```python
from build123d import *

# Parameters (mm, degrees)
F0_W      = 127
F0_H      = 76.2
F1_DEPTH  = 6.35
F3_DEPTH  = 6.35
F5_DEPTH  = 6.35
F7_DEPTH  = 6.35
F9_DEPTH  = 6.35
F11_DEPTH = 6.35
F13_DEPTH = 6.35


with BuildPart() as f1:
    # F0 (on Top) → F1 (new body)
    with BuildSketch(Plane.XY):
        with Locations((63.5, -38.1)):
            Rectangle(F0_W, F0_H)
    extrude(amount=F1_DEPTH)

    # F2 (on face) → F3 (cut, through all)
    with BuildSketch(Plane.XY.offset(6.35)):
        with BuildLine():
            ThreePointArc((8.986218, -38.1), (5.353199, -34.466981), (1.72018, -38.1))
            ThreePointArc((1.72018, -38.1), (5.353199, -41.733019), (8.986218, -38.1))
        make_face()
    extrude(amount=-F3_DEPTH, mode=Mode.SUBTRACT)

    # F4 (on face) → F5 (join)
    with BuildSketch(Plane.XY.offset(6.35)):
        with BuildLine():
            ThreePointArc((11.837447, -76.2), (35.286069, -38.1), (11.837447, 0))
            Line((11.837447, 0), (11.837447, -76.2))
        make_face()
    extrude(amount=F5_DEPTH)

    # F6 (on face) → F7 (cut)
    with BuildSketch(Plane.XY.offset(12.7)):
        with BuildLine():
            ThreePointArc((14.233802, -68.477303), (30.151871, -37.113268), (14.233802, -5.749233))
            Line((14.233802, -5.749233), (14.233802, -68.477303))
        make_face()
    extrude(amount=-F7_DEPTH, mode=Mode.SUBTRACT)

    # F8 (on face) → F9 (join)
    with BuildSketch(Plane.XY.offset(6.35)):
        Polygon((81.754573, -76.2), (51.588718, 0), (26.779415, -76.2), (36.64675, -76.2), (47.923706, -40.566836), (59.482586, -40.566836), (69.418724, -76.2), align=None)
        Polygon((45.034298, -35.888964), (51.588718, -15.757531), (59.341624, -35.888964), align=None, mode=Mode.SUBTRACT)
    extrude(amount=F9_DEPTH)

    # F10 (on face) → F11 (join)
    with BuildSketch(Plane.XY.offset(6.35)):
        with BuildLine():
            Line((84.432848, 0), (84.432848, -76.2))
            ThreePointArc((84.432848, -76.2), (115.125997, -38.1), (84.432848, 0))
        make_face()
        with BuildLine():
            Line((88.097863, -69.604993), (88.097863, -7.158854))
            ThreePointArc((88.097863, -7.158854), (109.621547, -38.381923), (88.097863, -69.604993))
        make_face(mode=Mode.SUBTRACT)
    extrude(amount=F11_DEPTH)

    # F12 (on face) → F13 (join)
    with BuildSketch(Plane.XY.offset(6.35)):
        with BuildLine():
            ThreePointArc((119.378194, -66.891998), (116.194297, -64.889157), (113.354176, -67.355387))
            Line((113.354176, -67.355387), (119.223736, -74.769571))
            Line((119.223736, -74.769571), (124.320991, -66.891998))
            ThreePointArc((124.320991, -66.891998), (121.849593, -64.724744), (119.378194, -66.891998))
        make_face()
    extrude(amount=F13_DEPTH)


solid = f1.part
```
Source: CAD feature listing. Evaluate the final solid. Frame: model axes, mm. A direction names the side the tool comes from. Coordinates: 2 decimals unless noted, no trailing zeros. Loops run counter-clockwise (first coordinate to the right, second up) from the corner with the lowest first, then second, coordinate; pieces in that order, holes last. Notation, with made-up numbers: (67.25, -30) -> (83.25, -30) arc R9 cw to (83.25, -25) -> close; hole circle Ø7 at (79.25, 86.5). An arc over 180 degrees is marked (long way). One line per item, written item: value. Start each with the question number.
Q1. Section query A-A, the plane y = -38.1. Return the cut outline in (x, z).
Q2. Line query: line 1 along X through (y, z) = (-38.1, 2); line 2 along X through (y, z) = (-59, 8.5); line 3 along X through (y, z) = (-30.5, 11). Output: solid intervals per line, ascending.
Q3. Mould query, pull axis Y, two halves, no side actions, for faces 5 (the face through (127, -39, 3)), 6 (the face through (63, 0, 3)), 7 (the face through (55.41, -25.68, 9.48)). Classes: pulls with the +Y half, pulls with the -Y half, needs draft (parallel to the pull), parting line crosses it, or undercut.
Q4. Section query B-B, the plane y = -59. Return the cut outline in (x, z).
Q5. Contact query for flat-ended pins moving along their axis: P1, Ø1.5, axis at y = -33, z = 8.5, coming from the -X side; P2, Ø9.5, axis at x = 5.5, y = -41, coming from the +Z side; P3, Ø1.9, axis at y = -27.5, z = 11, coming from the +X side. Output: stop coordinate, or through.
Q6. Section query C-C, the plane x = 106. Return the cut outline in (y, z).
Q7. Set-up query: faces 1 (the face through (11.837, -38, 9)), 2 (the face through (84.433, -38, 9)), 3 (the face through (66.88, -38.63, 9.48)), 4 (the face through (52, -30, 6.35)). Return all of +Z, -Z, +X, -X, +Y, -Y with unobstructed straight access to the full face (end or side cutting, diameter ignored); none if empty.
Q8. Section query D-D, the plane y = -28. Return the cut outline in (x, z).
Results:
1. outline: (0, 0) -> (1.72, 0) -> (1.72, 6.35) -> (0, 6.35) -> close; (8.99, 0) -> (127, 0) -> (127, 6.35) -> (115.13, 6.35) -> (115.13, 12.7) -> (109.62, 12.7) -> (109.62, 6.35) -> (88.1, 6.35) -> (88.1, 12.7) -> (84.43, 12.7) -> (84.43, 6.35) -> (66.67, 6.35) -> (66.67, 12.7) -> (39.18, 12.7) -> (39.18, 6.35) -> (35.29, 6.35) -> (35.29, 12.7) -> (30.14, 12.7) -> (30.14, 6.35) -> (14.23, 6.35) -> (14.23, 12.7) -> (11.84, 12.7) -> (11.84, 6.35) -> (8.99, 6.35) -> close
2. line 1: 0 to 1.72, 8.99 to 127
2. line 2: 11.84 to 14.23, 23.4 to 29.82, 32.38 to 42.09, 64.62 to 74.95, 84.43 to 88.1, 102.5 to 109.05
2. line 3: 11.84 to 14.23, 29.58 to 34.6, 41.66 to 46.79, 57.27 to 63.66, 84.43 to 88.1, 108.68 to 114.38
3. face 5: needs draft
3. face 6: pulls with the +Y half
3. face 7: undercut
4. outline: (0, 0) -> (127, 0) -> (127, 6.35) -> (109.05, 6.35) -> (109.05, 12.7) -> (102.5, 12.7) -> (102.5, 6.35) -> (88.1, 6.35) -> (88.1, 12.7) -> (84.43, 12.7) -> (84.43, 6.35) -> (74.95, 6.35) -> (74.95, 12.7) -> (64.62, 12.7) -> (64.62, 6.35) -> (42.09, 6.35) -> (42.09, 12.7) -> (32.38, 12.7) -> (32.38, 6.35) -> (29.82, 6.35) -> (29.82, 12.7) -> (23.4, 12.7) -> (23.4, 6.35) -> (14.23, 6.35) -> (14.23, 12.7) -> (11.84, 12.7) -> (11.84, 6.35) -> (0, 6.35) -> close
5. P1: x = 11.84
5. P2: z = 6.35
5. P3: x = 113.91
6. outline: (-76.2, 0) -> (0, 0) -> (0, 6.35) -> (-13.03, 6.35) -> (-13.03, 12.7) -> (-23.25, 12.7) -> (-23.25, 6.35) -> (-53.51, 6.35) -> (-53.51, 12.7) -> (-63.17, 12.7) -> (-63.17, 6.35) -> (-76.2, 6.35) -> close
7. face 1: +Z, -X, +Y, -Y
7. face 2: +Z, +Y, -Y
7. face 3: +Z, +Y
7. face 4: +Z
8. outline: (0, 0) -> (127, 0) -> (127, 6.35) -> (113.8, 6.35) -> (113.8, 12.7) -> (107.97, 12.7) -> (107.97, 6.35) -> (88.1, 6.35) -> (88.1, 12.7) -> (84.43, 12.7) -> (84.43, 6.35) -> (62.67, 6.35) -> (62.67, 12.7) -> (56.3, 12.7) -> (56.3, 6.35) -> (47.6, 6.35) -> (47.6, 12.7) -> (42.47, 12.7) -> (42.47, 6.35) -> (34.07, 6.35) -> (34.07, 12.7) -> (29.07, 12.7) -> (29.07, 6.35) -> (14.23, 6.35) -> (14.23, 12.7) -> (11.84, 12.7) -> (11.84, 6.35) -> (0, 6.35) -> close
